from build123d import *

# Parameters (mm, degrees)
SKETCH_1_W          = 15
SKETCH_1_H          = 15
SKETCH_1_W_2        = 13
SKETCH_1_H_2        = 13
EXTRUDE_1_DEPTH     = 187.2
SKETCH_2_R          = 2
CUT_EXTRUDE_1_DEPTH = 188.949700718
SKETCH_3_R          = 2
CUT_EXTRUDE_2_DEPTH = 188.949700718


with BuildPart() as part:
    # ｽｹｯﾁ1 → 押し出し-薄板1 (new body)
    with BuildSketch(Plane(origin=(0, 0, 0), x_dir=(0, 0, -1), z_dir=(1, 0, 0))):
        Rectangle(SKETCH_1_W, SKETCH_1_H)
        Rectangle(SKETCH_1_W_2, SKETCH_1_H_2, mode=Mode.SUBTRACT)
    extrude(amount=EXTRUDE_1_DEPTH)

    # ｽｹｯﾁ2 → ｶｯﾄ - 押し出し1 (cut, through all)
    with BuildSketch(Plane.XY.offset(7.5)):
        with Locations((7.5, 0)):
            Circle(SKETCH_2_R)
        with Locations((47.5, 0)):
            Circle(SKETCH_2_R)
        with Locations(Location((139.7, 0, 0), (0, 0, 180))):
            Circle(SKETCH_2_R)
        with Locations(Location((179.7, 0, 0), (0, 0, 180))):
            Circle(SKETCH_2_R)
    extrude(amount=-CUT_EXTRUDE_1_DEPTH, mode=Mode.SUBTRACT)

    # ｽｹｯﾁ3 → ｶｯﾄ - 押し出し2 (cut, through all)
    with BuildSketch(Plane(origin=(0, 7.5, 0), x_dir=(1, 0, 0), z_dir=(0, 1, 0))):
        with Locations(Location((58.6, 0, 0), (0, 0, 270))):
            Circle(SKETCH_3_R)
        with Locations(Location((128.6, 0, 0), (0, 0, 270))):
            Circle(SKETCH_3_R)
    extrude(amount=-CUT_EXTRUDE_2_DEPTH, mode=Mode.SUBTRACT)


solid = part.part
Input: part model. Units: mm. Frame: model coordinates. A direction names the side the tool comes from. Give positions to 0.01 mm unless a question says otherwise; leave off trailing zeros. Loops run counter-clockwise (first coordinate to the right, second up) from the corner with the lowest first, then second, coordinate; pieces in that order, holes last. Notation, with made-up numbers: (27.5, 5.25) -> (78.5, 5.25) arc R19 cw to (78.5, 20.25) -> close; hole circle Ø3 at (34.25, 34.5). An arc over 180 degrees is marked (long way). Answer as a JSON object with one key per item and string values. Group by question number.
Item 1: Line query: probe 1 along X at (y, z) = (7.3, 0); probe 2 along Z at (x, y) = (37.5, 0). Output: solid intervals per line, ascending.
Item 2: Reachability of faces 5 (the flat face through (92, -6.5, 0)), 6 (the flat face through (187.2, 0, 7)) from +Z, -Z, +X, -X, +Y, -Y: full face, straight path, thin tool, end or side. Return the list, or none.
Item 3: Cut plane C-C, the plane x = 63. Return the cut outline in (y, z).
Item 4: Cut plane A-A, the plane y = 4. Return the cut outline in (x, z), and give its area (3 significant figures).
Item 5: Cut plane B-B, the plane x = 128.6. Return the cut outline in (y, z).
Item 6: Pull-direction query (Y, two-part tool) for faces 1 (the flat face through (92, -7.5, 0)), 2 (the flat face through (92, 0, 7.5)), 3 (the flat face through (92, 7.5, 0)), 4 (the flat face through (92, 6.5, 0)); classes: released by +Y, released by -Y, zero draft, split by the parting line, or undercut.
Checks:
{
 "1": {"probe 1": "x = 0 to 56.6, 60.6 to 126.6, 130.6 to 187.2", "probe 2": "z = -7.5 to -6.5, 6.5 to 7.5"},
 "2": {"face 5": "+X, -X", "face 6": "+Z, -Z, +X, +Y, -Y"},
 "3": {"outline": "(-7.5, -7.5) -> (7.5, -7.5) -> (7.5, 7.5) -> (-7.5, 7.5) -> close; hole (-6.5, -6.5) -> (6.5, -6.5) -> (6.5, 6.5) -> (-6.5, 6.5) -> close"},
 "4": {"outline": "(0, -7.5) -> (187.2, -7.5) -> (187.2, -6.5) -> (0, -6.5) -> close; (0, 6.5) -> (187.2, 6.5) -> (187.2, 7.5) -> (0, 7.5) -> close", "area": "374 mm²"},
 "5": {"outline": "(-7.5, -7.5) -> (7.5, -7.5) -> (7.5, -2) -> (6.5, -2) -> (6.5, -6.5) -> (-6.5, -6.5) -> (-6.5, -2) -> (-7.5, -2) -> close; (-7.5, 2) -> (-6.5, 2) -> (-6.5, 6.5) -> (6.5, 6.5) -> (6.5, 2) -> (7.5, 2) -> (7.5, 7.5) -> (-7.5, 7.5) -> close"},
 "6": {"face 1": "released by -Y", "face 2": "zero draft", "face 3": "released by +Y", "face 4": "undercut"}
}
